Drawing for the job (mm, zero at the part's lowest x, y, z). Give positions to 0.01 mm unless a question says otherwise; leave off trailing zeros. Loops run counter-clockwise (first coordinate to the right, second up) from the corner with the lowest first, then second, coordinate; pieces in that order, holes last. Notation, with made-up numbers: (89, 76) -> (111, 76) arc R33 cw to (111, 112) -> close; hole circle Ø8 at (75.25, -12.5). An arc over 180 degrees is marked (long way). Write item = value, one per line.
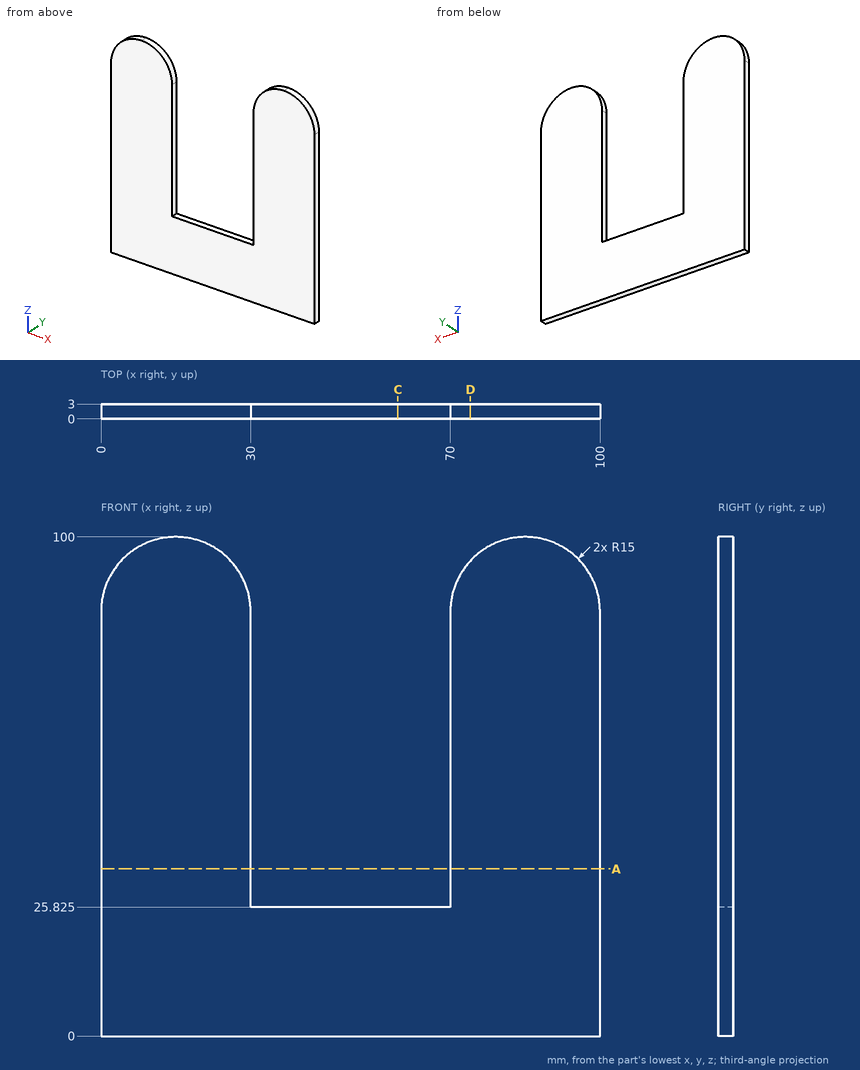
1) Slice it at D-D, the plane x = 74. List the corners of the cut face in (y, z), and give its area (3 significant figures).
Resolved:
outline = (0, 0) -> (3, 0) -> (3, 95.2) -> (0, 95.2) -> close
area = 286 mm²
2) Drill centre lines: line 1 along X through (y, z) = (0.55, 28); line 2 along Z through (x, y) = (84.5, 1.35); line 3 along Z through (x, y) = (32.5, 0.25) (3 decimals). Where is each one in solid material? Low to high. Write a range as [from, to].
Resolved:
line_1 = [0, 30], [70, 100]
line_2 = [0, 99.99]
line_3 = [0, 25.825]
3) Slice it at A-A, the plane z = 33.5. List the corners of the cut face in (x, y).
Resolved:
outline = (0, 0) -> (30, 0) -> (30, 3) -> (0, 3) -> close; (70, 0) -> (100, 0) -> (100, 3) -> (70, 3) -> close
4) Slice it at C-C, the plane x = 59.5. List the corners of the cut face in (y, z) (3 decimals), and give its area (3 significant figures).
Resolved:
outline = (0, 0) -> (3, 0) -> (3, 25.825) -> (0, 25.825) -> close
area = 77.5 mm²
5) Drop flat-ended pins along their axis: P1, Ø5, axis at x = 57, z = 22.5, coming from the -Y side; P2, Ø1.5, axis at x = 40.5, y = 1.5, coming from the +Z side (3 decimals). Give the stop position or say it passes through.
Resolved:
P1 = 0
P2 = 25.825
